Here's how the part is built. I have some questions about the finished solid (model axes, mm). Face numbers are marked on the shaded views. A direction names the side the tool comes from. Coordinates: 2 decimals unless noted, no trailing zeros. Write each loop counter-clockwise with the first axis right and the second up, starting at its lowest first coordinate (ties: lowest second). Pieces come first, ordered by that corner, then holes. Notation, with made-up numbers: (62.5, -10.5) -> (66.5, -10.5) arc R32 ccw to (66.5, 23.5) -> close; hole circle Ø5 at (-8, 51.5). An arc over 180 degrees is marked (long way). Put each result on its own line as item: value. Start each with the question number.
Item 1: I want a section at C-C, the plane z = 6. List the corners of the cut face in (x, y) for me.
Item 2: I need wall thicknesses on line 1 (Z direction, x = 0, y = 4.5); line 2 (Y direction, x = 0, z = -6.25). Which ranges of each line are inside material? Lowest first, please. Write a range as [from, to].
Item 3: I want a section at B-B, the plane y = 14.5. List the corners of the cut face in (x, z) for me, then the cut area to 3 significant figures.
Item 4: On a 3-axis mill with a long thin cutter (end or side, diameter ignored), from which of +Z, -Z, +X, -X, +Y, -Y can I reach the whole of each face in a straight line? I mean the marked faces 4, 5, 6, 7 and 8. Say none if no direction works.
Item 5: I want a section at D-D, the plane y = 18. List the corners of the cut face in (x, z) for me, then the cut area to 3 significant figures.
Item 6: I want a section at A-A, the plane z = 0. List the corners of the cut face in (x, y) for me.
Item 7: If we mould it in two halves opening along X, with no side actions, what happens to the marked faces 1, 2 and 3? For each: released by +X, released by -X, zero draft, split by the parting line, or undercut.
Item 8: For pin 1 (3 mm diameter, centred on y = 16, z = 6.5, fed in from -X); pin 2 (6.5 mm diameter, centred on x = -4.5, z = 0.5, fed in from +Y); pin 3 (1 mm diameter, centred on x = -1.5, z = 2, fed in from -Y); pin 4 (1.1 mm diameter, centred on y = 13, z = -5.5, fed in from +X), each with a flat end and sliding along its axis, tell me the tip position at first contact or that it passes through.
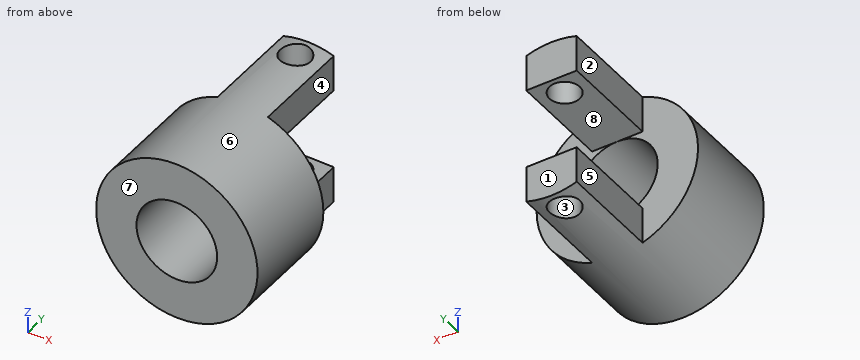
from build123d import *

# Parameters (mm, degrees)
SKETCH_1_R               = 8
EXTRUDE_1_DEPTH          = 20
CUT_EXTRUDE_1_DEPTH      = 23.978250586
CUT_EXTRUDE_1_DEPTH_BACK = 23.978250586
SKETCH_2_W               = 5.5
SKETCH_2_H               = 10
CUT_EXTRUDE_2_DEPTH      = 24.963513933
CUT_EXTRUDE_2_DEPTH_BACK = 24.963513933
SKETCH_3_W               = 8
SKETCH_3_H               = 10
CUT_EXTRUDE_3_DEPTH      = 23.978250586
CUT_EXTRUDE_3_DEPTH_BACK = 23.978250586
SKETCH_4_R               = 1.5
CUT_EXTRUDE_4_DEPTH      = 23.978250743
CUT_EXTRUDE_4_DEPTH_BACK = 23.978250743
SKETCH_5_R               = 4


with BuildPart() as part:
    # 草图1 → 凸台-拉伸1 (new body)
    with BuildSketch(Plane(origin=(0, 0, 0), x_dir=(1, 0, 0), z_dir=(0, 1, 0))):
        with Locations(Location((0, 0, 0), (0, 0, 270))):
            Circle(SKETCH_1_R)
    extrude(amount=EXTRUDE_1_DEPTH)

    # 草图2 → 切除-拉伸1 (cut, two sides: drawn at the far end of the back side and taken through both)
    with BuildSketch(Plane.XY.offset(-CUT_EXTRUDE_1_DEPTH_BACK)):
        with Locations((-5.25, 15)):
            Rectangle(SKETCH_2_W, SKETCH_2_H)
        with Locations((5.25, 15)):
            Rectangle(SKETCH_2_W, SKETCH_2_H)
    extrude(amount=CUT_EXTRUDE_1_DEPTH + CUT_EXTRUDE_1_DEPTH_BACK, mode=Mode.SUBTRACT)

    # 草图3 → 切除-拉伸2 (cut, two sides: drawn at the far end of the back side and taken through both)
    with BuildSketch(Plane.ZY.offset(2.5).offset(-CUT_EXTRUDE_2_DEPTH_BACK)):
        with Locations((0, 15)):
            Rectangle(SKETCH_3_W, SKETCH_3_H)
    extrude(amount=CUT_EXTRUDE_2_DEPTH + CUT_EXTRUDE_2_DEPTH_BACK, mode=Mode.SUBTRACT)

    # 草图4 → 切除-拉伸3 (cut, two sides: drawn at the far end of the back side and taken through both)
    with BuildSketch(Plane.XY.offset(-CUT_EXTRUDE_3_DEPTH_BACK)):
        with Locations((0, 18)):
            Circle(SKETCH_4_R)
    extrude(amount=CUT_EXTRUDE_3_DEPTH + CUT_EXTRUDE_3_DEPTH_BACK, mode=Mode.SUBTRACT)

    # 草图5 → 切除-拉伸4 (cut, two sides: drawn at the far end of the back side and taken through both)
    with BuildSketch(Plane.XZ.offset(-CUT_EXTRUDE_4_DEPTH_BACK)):
        with Locations(Location((0, 0, 0), (0, 0, 270))):
            Circle(SKETCH_5_R)
    extrude(amount=CUT_EXTRUDE_4_DEPTH + CUT_EXTRUDE_4_DEPTH_BACK, mode=Mode.SUBTRACT)


solid = part.part
Calculated:
1. outline: (-5.29, 0) -> (5.29, 0) -> (5.29, 10) -> (2.5, 10) -> (2.5, 20) -> (-2.5, 20) -> (-2.5, 10) -> (-5.29, 10) -> close; hole circle Ø3 at (0, 18)
2. line 1: z = [-8, -4], [4, 8]
2. line 2: y = [0, 16.5], [19.5, 20]
3. outline: (-2.5, -7.6) arc R8 ccw to (2.5, -7.6) -> (2.5, -4) -> (-2.5, -4) -> close; (-2.5, 4) -> (2.5, 4) -> (2.5, 7.6) arc R8 ccw to (-2.5, 7.6) -> close
3. area: 38.7 mm2
4. face 4: +Z, -Z, +X, +Y
4. face 5: +Z, -Z, -X, +Y
4. face 6: +Y, -Y
4. face 7: +Z, -Z, +X, -X, -Y
4. face 8: +X, -X, +Y
5. outline: (-2.5, -7.6) arc R8 ccw to (-1.5, -7.86) -> (-1.5, -4) -> (-2.5, -4) -> close; (-2.5, 4) -> (-1.5, 4) -> (-1.5, 7.86) arc R8 ccw to (-2.5, 7.6) -> close; (1.5, -7.86) arc R8 ccw to (2.5, -7.6) -> (2.5, -4) -> (1.5, -4) -> close; (1.5, 4) -> (2.5, 4) -> (2.5, 7.6) arc R8 ccw to (1.5, 7.86) -> close
5. area: 15.0 mm2
6. outline: (-8, 0) -> (-4, 0) -> (-4, 10) -> (-8, 10) -> close; (4, 0) -> (8, 0) -> (8, 10) -> (4, 10) -> close
7. face 1: zero draft
7. face 2: released by -X
7. face 3: undercut
8. pin 1: stops at x = -2.5
8. pin 2: stops at y = 10
8. pin 3: passes through
8. pin 4: stops at x = 2.5
